Job drawing, mm, ordinate dimensions from the low corner. One solid piece. A direction names the side the tool comes from. Give positions to 0.01 mm unless a question says otherwise; leave off trailing zeros.
Item 1: Flat gauge pins, fed straight in: P1, Ø5, axis at x = 67.5, y = 36, coming from the -Z side (1 decimal); P2, Ø8.5, axis at y = 11.5, z = 72.5, coming from the +X side; P3, Ø1.4, axis at y = 23, z = 30.5, coming from the -X side. Where does each tip first touch, or does it go through?
Item 2: Which spindle directions (+Z, -Z, +X, -X, +Y, -Y) get a long thin tool onto all of the face, cutting with end or side? Do the marked faces 1, 2, 3, 4 and 5. Say none if no direction does.
Item 3: Two-plate mould, pull along X, no slides. Class the marked faces 6, 7 and 8: released by +X, released by -X, zero draft, split by the parting line, or undercut.
Item 4: Wall check: L1, parallel to Z at x = 63.5, y = 15 (1 decimal); L2, parallel to Z at x = 25, y = 36; L3, parallel to Z at x = 73.5, y = 24. Give the ranges that are in metal, low to high.
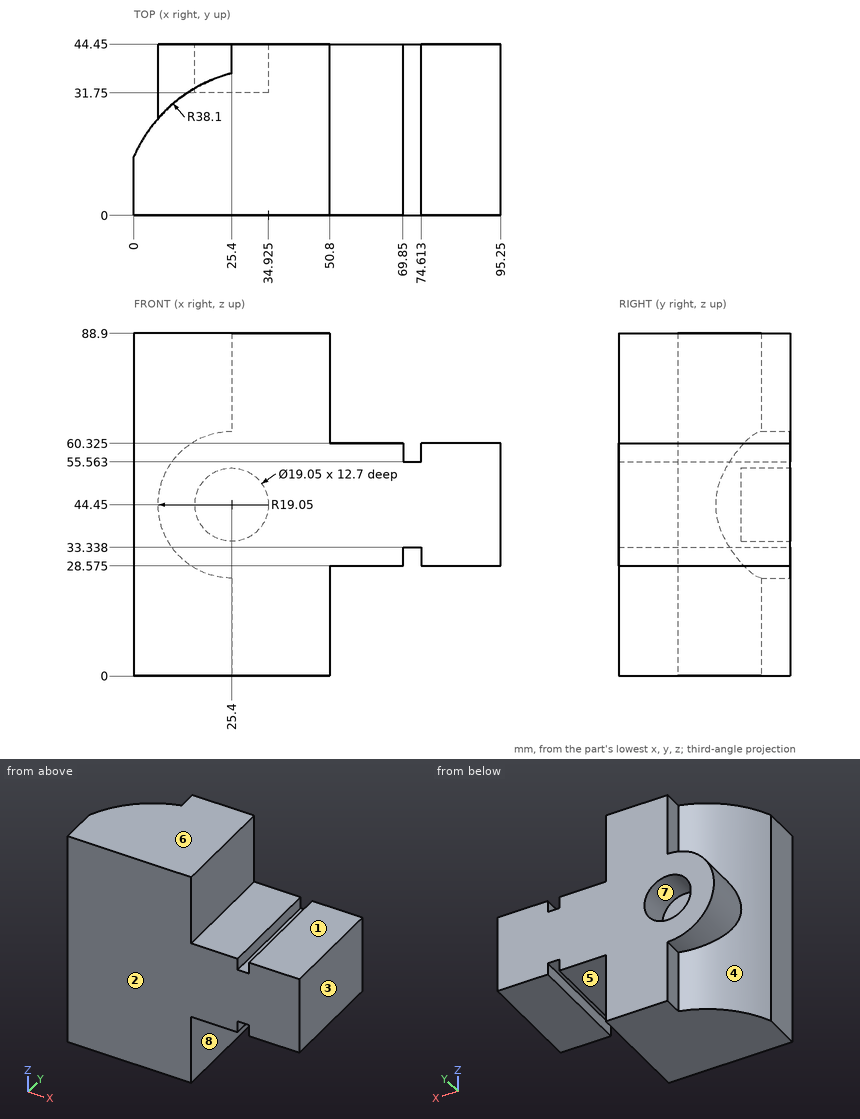
The answers:
1. P1: stops at z = 28.6
1. P2: stops at x = 50.8
1. P3: stops at x = 4.03
2. face 1: +Z, +X, +Y, -Y
2. face 2: +Z, -Z, +X, -X, -Y
2. face 3: +Z, -Z, +X, +Y, -Y
2. face 4: -X, +Y
2. face 5: -Z, +X, +Y, -Y
3. face 6: zero draft
3. face 7: undercut
3. face 8: released by +X
4. L1: z = 28.6 to 60.3
4. L2: z = 0 to 34.93, 53.97 to 88.9
4. L3: z = 33.34 to 55.56
